```python
from build123d import *

# Parameters (mm, degrees)
SKETCH_1_W               = 170
SKETCH_1_H               = 76
EXTRUDE_1_DEPTH          = 3.5
FILLET_1_R               = 10
SKETCH_2_W               = 8
SKETCH_2_H               = 20
CUT_EXTRUDE_1_DEPTH      = 3
SKETCH_3_W               = 8
SKETCH_3_H               = 20
CUT_EXTRUDE_2_DEPTH      = 3
SKETCH_6_R               = 1.8
CUT_EXTRUDE_4_DEPTH      = 4
MIRROR_2_COPY_1_SKETCH_R = 1.8
MIRROR_2_COPY_1_DEPTH    = 4


with BuildPart() as part:
    # 草图1 → 凸台-拉伸1 (new body)
    with BuildSketch(Plane.XY):
        Rectangle(SKETCH_1_W, SKETCH_1_H)
    extrude(amount=EXTRUDE_1_DEPTH)

    # 圆角1
    fillet_1_edges = [part.edges().sort_by_distance(p)[0] for p in [
        (85, -38, 1.75),
        (-85, -38, 1.75),
        (-85, 38, 1.75),
        (85, 38, 1.75),
    ]]
    fillet(fillet_1_edges, radius=FILLET_1_R)

    # 草图2 → 切除-拉伸1 (cut)
    with BuildSketch(Plane(origin=(0, 0, 0), x_dir=(-1, 0, 0), z_dir=(0, 0, -1))):
        with Locations((-27, 0)):
            Rectangle(SKETCH_2_W, SKETCH_2_H)
    extrude(amount=-CUT_EXTRUDE_1_DEPTH, mode=Mode.SUBTRACT)

    # 草图3 → 切除-拉伸2 (cut)
    with BuildSketch(Plane(origin=(0, 0, 0), x_dir=(-1, 0, 0), z_dir=(0, 0, -1))):
        with Locations((71, 0)):
            Rectangle(SKETCH_3_W, SKETCH_3_H)
    extrude(amount=-CUT_EXTRUDE_2_DEPTH, mode=Mode.SUBTRACT)

    # 草图6 → 切除-拉伸4 (cut)
    with BuildSketch(Plane(origin=(0, 0, 0), x_dir=(-1, 0, 0), z_dir=(0, 0, -1))):
        with Locations((71, -19)):
            Circle(SKETCH_6_R)
    cut_extrude_4 = extrude(amount=-CUT_EXTRUDE_4_DEPTH, mode=Mode.SUBTRACT)

    # 镜向1: 切除-拉伸4 across plane
    add(cut_extrude_4.mirror(Plane.ZX), mode=Mode.SUBTRACT)

    # 镜向2: 切除-拉伸4 across plane
    add(cut_extrude_4.mirror(Plane(origin=(-22, 0, 0), x_dir=(0, 0, 1), z_dir=(1, 0, 0))), mode=Mode.SUBTRACT)

    # 镜向2 copy 1 sketch → 镜向2 copy 1 (cut)
    with BuildSketch(Plane(origin=(-44, 0, 0), x_dir=(1, 0, 0), z_dir=(0, 0, -1))):
        with Locations((71, -19)):
            Circle(MIRROR_2_COPY_1_SKETCH_R)
    extrude(amount=-MIRROR_2_COPY_1_DEPTH, mode=Mode.SUBTRACT)


solid = part.part
```
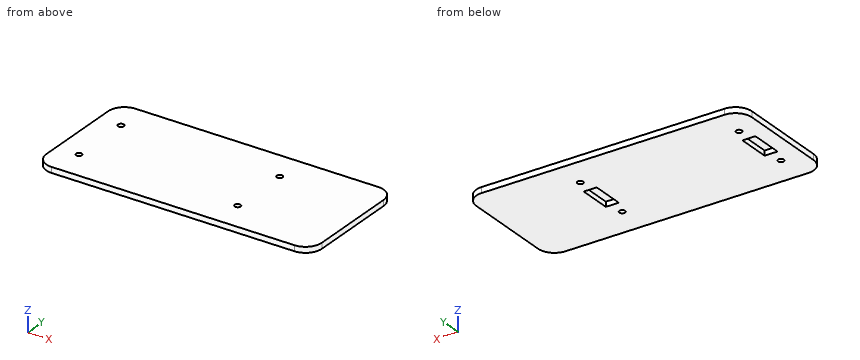
Check sheet for the modelled part. Datum: model origin and axes. Units: mm. Coordinates: 2 decimals unless noted, no trailing zeros. Order: outer loops, then holes, each group sorted by start corner. A loop starts at its lowest first (then second) coordinate and runs counter-clockwise, first axis right, second up. Notation, with made-up numbers: M -5.5,-33 L 11.5,-33 A26 ccw 11.5,6 Z; hole C 65,81 d2. An arc over 180 degrees is marked long. One line per question, with ' | ' between items. Start each with the question number.
Item 1: Sectioned sample at A-A on z = 1.95. Record the cut outline in (x, y).
Item 2: Sectioned sample at B-B on x = 27. Record the cut outline in (y, z).
Item 3: Material ranges on line 1 (Y direction, x = -71, z = 1.3); line 2 (X direction, y = -7, z = 2.65); line 3 (X direction, y = 19, z = 2.3), recorded low to high.
Item 4: Gauge pin test, flat ends, axial feed: P1, Ø4, axis at x = 27.5, y = -2, coming from the -Z side; P2, Ø3, axis at x = 27, y = 19, coming from the +Z side; P3, Ø2, axis at y = 29.5, z = 1, coming from the +X side. Record the tip position at first contact, or that the pin passes through.
Item 5: Sectioned sample at C-C on y = -19. Record the cut outline in (x, z), and give its area (3 significant figures).
Answer below:
1) outline: M -85,-28 A10 ccw -75,-38 L 75,-38 A10 ccw 85,-28 L 85,28 A10 ccw 75,38 L -75,38 A10 ccw -85,28 Z; hole M -75,-10 L -67,-10 L -67,10 L -75,10 Z; hole C -71,-19 d3.6; hole C -71,19 d3.6; hole M 23,-10 L 31,-10 L 31,10 L 23,10 Z; hole C 27,-19 d3.6; hole C 27,19 d3.6
2) outline: M -38,0 L -20.8,0 L -20.8,3.5 L -38,3.5 Z; M -17.2,0 L -10,0 L -10,3 L 10,3 L 10,0 L 17.2,0 L 17.2,3.5 L -17.2,3.5 Z; M 20.8,0 L 38,0 L 38,3.5 L 20.8,3.5 Z
3) line 1: y = -38 to -20.8, -17.2 to -10, 10 to 17.2, 20.8 to 38 | line 2: x = -85 to -75, -67 to 23, 31 to 85 | line 3: x = -85 to -72.8, -69.2 to 25.2, 28.8 to 85
4) P1: stops at z = 3 | P2: passes through | P3: stops at x = 84.99
5) outline: M -85,0 L -72.8,0 L -72.8,3.5 L -85,3.5 Z; M -69.2,0 L 25.2,0 L 25.2,3.5 L -69.2,3.5 Z; M 28.8,0 L 85,0 L 85,3.5 L 28.8,3.5 Z | area: 570 mm^2
